Here's how the part is built. I have some questions about the finished solid (model axes, mm). A direction names the side the tool comes from. Round coordinates to 2 decimals unless told otherwise and drop trailing zeros. Write each loop counter-clockwise with the first axis right and the second up, starting at its lowest first coordinate (ties: lowest second). Pieces come first, ordered by that corner, then holes. Notation, with made-up numbers: (74.5, -28.75) - (127.5, -28.75) arc R6 cw to (127.5, -19.75) - close; hole circle Ø11 at (71.5, 18). An arc over 180 degrees is marked (long way). Use one line per item in the form item = value. Start each with the question number.
1. We'd pull the mould along X, two halves only. Please class faces 5 (the flat face through (-96, -32.999, 2)), 6 (the flat face through (46.402, -18, 2)), 7 (the flat face through (-9.098, -40, 2)): +X half, -X half, draft (parallel to the pull), parting line (faces both ways), or undercut.
2. I want a section at A-A, the plane y = -24.25. List the corners of the cut face in (x, z) for me.
3. Will these pins go through, and if not, where does the flat tip stop? pin 1 (3 mm diameter, centred on x = 27, z = 1.5, fed in from +Y); pin 2 (2.5 mm diameter, centred on y = -41.5, z = 2, fed in from +X); pin 3 (8 mm diameter, centred on x = -53.5, y = -39.5, fed in from -Z).
4. If I drill on line 1 along X through (y, z) = (-32, 4.5); line 2 along X through (y, z) = (-39.5, 4.2); line 3 along Y through (x, z) = (-24, 1.05), over which ranges is the centre line in solid material (lowest first)?
5. I want a section at C-C, the plane z = 1.9. State how many separate pieces and enclosed holes the cut face has, plus the area to 3 significant figures.
6. Which directions (+Z, -Z, +X, -X, +Y, -Y) give clear straight access to the entire face, cutting with the end or side of a thin tool? Please do faces 1 (the flat face through (-53.098, -40, 2)), 2 (the flat face through (-24, -32.999, 2)), 3 (the flat face through (-2, -17.999, 2)), 4 (the flat face through (49, -22.999, 2)).
7. I want a section at D-D, the plane y = -35. List the corners of the cut face in (x, z) for me.
8. I want a section at B-B, the plane x = 24.5. List the corners of the cut face in (y, z) for me, plus the area to 3 significant figures.
```python
from build123d import *

# Parameters (mm, degrees)
SKETCH1_W           = 5
SKETCH1_H           = 10
BOSS_EXTRUDE1_DEPTH = 5


with BuildPart() as part:
    # Sketch1 → Boss-Extrude1 (new body)
    with BuildSketch(Plane.XY):
        Polygon((46.402376673, -17.999000463), (46.402376673, -22.999000463), (51.402376673, -22.999000463), (51.402376673, -32.999000463), (46.402376673, -32.999000463), (46.402376673, -37.999000463), (46.402376673, -42.999000463), (35.902376673, -42.999000463), (35.902376673, -37.999000463), (20.902376673, -37.999000463), (20.902376673, -42.999000463), (5.902376673, -42.999000463), (5.902376673, -37.999000463), (-9.097623327, -37.999000463), (-9.097623327, -42.999000463), (-38.097623327, -42.999000463), (-38.097623327, -37.999000463), (-53.097623327, -37.999000463), (-53.097623327, -42.999000463), (-68.097623327, -42.999000463), (-68.097623327, -37.999000463), (-83.097623327, -37.999000463), (-83.097623327, -42.999000463), (-93.597623327, -42.999000463), (-93.597623327, -37.999000463), (-93.597623327, -32.999000463), (-98.597623326, -32.999000463), (-98.597623326, -22.999000463), (-93.597623327, -22.999000463), (-93.597623327, -17.999000463), (-93.597623327, -12.999000463), (-83.097623327, -12.999000463), (-83.097623327, -17.999000463), (-68.097623327, -17.999000463), (-68.097623327, -12.999000463), (-53.097623327, -12.999000463), (-53.097623327, -17.999000463), (-38.097623327, -17.999000463), (-38.097623327, -12.999000463), (-9.097623327, -12.999000463), (-9.097623327, -17.999000463), (5.902376673, -17.999000463), (5.902376673, -12.999000463), (20.902376673, -12.999000463), (20.902376673, -17.999000463), (35.902376673, -17.999000463), (35.902376673, -12.999000463), (46.402376673, -12.999000463), align=None)
        with Locations((11.402376673, -27.999000463)):
            Rectangle(SKETCH1_W, SKETCH1_H, mode=Mode.SUBTRACT)
        with Locations((-23.597623327, -27.999000463)):
            Rectangle(SKETCH1_W, SKETCH1_H, mode=Mode.SUBTRACT)
        with Locations((-58.597623327, -27.999000463)):
            Rectangle(SKETCH1_W, SKETCH1_H, mode=Mode.SUBTRACT)
    extrude(amount=BOSS_EXTRUDE1_DEPTH)


solid = part.part
```
Model answer:
q1.face_5 = draft
q1.face_6 = +X half
q1.face_7 = undercut
q2.outline = (-98.6, 0) - (-61.1, 0) - (-61.1, 5) - (-98.6, 5) - close; (-56.1, 0) - (-26.1, 0) - (-26.1, 5) - (-56.1, 5) - close; (-21.1, 0) - (8.9, 0) - (8.9, 5) - (-21.1, 5) - close; (13.9, 0) - (51.4, 0) - (51.4, 5) - (13.9, 5) - close
q3.pin_1 = -18
q3.pin_2 = 46.4
q3.pin_3 = 0
q4.line_1 = -98.6 to -61.1, -56.1 to -26.1, -21.1 to 8.9, 13.9 to 51.4
q4.line_2 = -93.6 to -83.1, -68.1 to -53.1, -38.1 to -9.1, 5.9 to 20.9, 35.9 to 46.4
q4.line_3 = -43 to -33, -23 to -13
q5.separate_pieces = 1
q5.enclosed_holes = 3
q5.area = 3,550 mm2
q6.face_1 = +Z, -Z, -Y
q6.face_2 = +Z, -Z
q6.face_3 = +Z, -Z, +Y
q6.face_4 = +Z, -Z, +X, +Y
q7.outline = (-93.6, 0) - (46.4, 0) - (46.4, 5) - (-93.6, 5) - close
q8.outline = (-38, 0) - (-18, 0) - (-18, 5) - (-38, 5) - close
q8.area = 100 mm2
